```python
from build123d import *

# Parameters (mm, degrees)
F1_DEPTH = 75
F3_D     = 8
F3_DEPTH = 20
F3_TIP   = 2.4034424761


with BuildPart() as f1:
    # F0 (on Front) → F1 (new body)
    with BuildSketch(Plane.XZ):
        Polygon((-31.7075045779, 35.5722052749), (-41.7075045779, 35.5722052749), (-41.7075045779, -124.4277947251), (3.2924954221, -124.4277947251), align=None)
    extrude(amount=F1_DEPTH)

    # F3
    with Locations(Plane.XZ.offset(75)):
        with Locations((-26.7075045779, -64.4277947251), (-26.7075045779, -104.4277947251)):
            Hole(F3_D / 2, depth=F3_DEPTH)
            with Locations((0, 0, -(F3_DEPTH + F3_TIP / 2))):  # 118° drill point
                Cone(0, F3_D / 2, F3_TIP, mode=Mode.SUBTRACT)


solid = f1.part
```
For this review, take the finished solid that the model builds, in its own axes (mm). A direction names the side the tool comes from. Coordinates: 2 decimals unless noted, no trailing zeros. Loops run counter-clockwise (first coordinate to the right, second up) from the corner with the lowest first, then second, coordinate; pieces in that order, holes last. Notation, with made-up numbers: (1.25, 52.5) -> (29.25, 52.5) arc R25 cw to (29.25, 70.5) -> close; hole circle Ø8 at (-24, 52). An arc over 180 degrees is marked (long way). Return JSON: item names as keys, results as strings. Group by question number.
(1) For pin 1 Ø8 at (x, z) = (-27.5, -5.5) entering from +Y; pin 2 Ø7 at (x, z) = (-26.71, -64.43) entering from -Y; pin 3 Ø12 at (y, z) = (-37.5, 19) entering from +X, all flat-tipped, find the tip position at first contact; note any pin that passes through.
(2) Consider section A-A, the plane y = -68. Give the boundary of the cut face in (x, z), plus the area to 3 significant figures.
(3) Mouldability with a two-part tool opening along X and no side actions: class faces 3 (the cylindrical face through (-30.523, -64.86, -103.226)), 4 (the flat face through (-41.708, -37, -43)), 5 (the flat face through (-20, -37, -124.428)), 6 (the flat face through (-13.96, -36.98, -45.55)) as pulls with the +X half, pulls with the -X half, needs draft (parallel to the pull), parting line crosses it, or undercut.
(4) To check wall thickness, follow L1, parallel to X at y = -25, z = -69.5; L2, parallel to X at y = -5, z = -51. State the ranges of each line that lie inside material, in increasing order.
(5) Consider section C-C, the plane z = -84.5. Give the boundary of the cut face in (x, y), plus the area to 3 significant figures.
(6) Tool access review of faces 1 (the flat face through (-25, 0, -61)), 2 (the cylindrical face through (-28.858, -64.86, -61.055)): name each direction out of +Z, -Z, +X, -X, +Y, -Y from which nothing blocks a thin tool from reaching the whole face with its end or side.
(7) Consider section B-B, the plane y = -49. Give the boundary of the cut face in (x, z).
Results below:
{
 "1": {"pin 1": "stops at y = 0", "pin 2": "stops at y = -54.7", "pin 3": "stops at x = -26.77"},
 "2": {"outline": "(-41.71, -124.43) -> (3.29, -124.43) -> (-31.71, 35.57) -> (-41.71, 35.57) -> close; hole circle Ø8 at (-26.71, -104.43); hole circle Ø8 at (-26.71, -64.43)", "area": "4,300 mm2"},
 "3": {"face 3": "undercut", "face 4": "pulls with the -X half", "face 5": "needs draft", "face 6": "pulls with the +X half"},
 "4": {"L1": "x = -41.71 to -8.72", "L2": "x = -41.71 to -12.77"},
 "5": {"outline": "(-41.71, -75) -> (-5.44, -75) -> (-5.44, 0) -> (-41.71, 0) -> close", "area": "2,720 mm2"},
 "6": {"face 1": "+Z, -Z, +X, -X, +Y", "face 2": "-Y"},
 "7": {"outline": "(-41.71, -124.43) -> (3.29, -124.43) -> (-31.71, 35.57) -> (-41.71, 35.57) -> close"}
}
